from build123d import *

# Parameters (mm, degrees)
BOSS_EXTRUDE1_DEPTH = 15
BOSS_EXTRUDE2_DEPTH = 60
SKETCH3_W           = 30
SKETCH3_H           = 17.5
SKETCH3_H_2         = 34.418211048
CUT_EXTRUDE1_DEPTH  = 199.997487421
BOSS_EXTRUDE3_START = -45
SKETCH4_R           = 5
BOSS_EXTRUDE3_DEPTH = 30


with BuildPart() as part:
    # Sketch1 → Boss-Extrude1 (new body)
    with BuildSketch(Plane(origin=(0, 0, 0), x_dir=(1, 0, 0), z_dir=(0, 1, 0))):
        with BuildLine():
            Line((0, 0), (150, 0))
            Line((150, 0), (150, 60))
            Line((150, 60), (0, 60))
            ThreePointArc((0, 60), (-30, 30), (0, 0))
        make_face()
    extrude(amount=BOSS_EXTRUDE1_DEPTH)

    # Sketch2 → Boss-Extrude2 (add)
    with BuildSketch(Plane.XY):
        with BuildLine():
            Line((60, 15), (90, 15))
            Line((90, 15), (90, 45))
            ThreePointArc((90, 45), (75, 60), (60, 45))
            Line((60, 45), (60, 15))
        make_face()
        with BuildLine():
            Line((120, 15), (150, 15))
            Line((150, 15), (150, 35))
            ThreePointArc((150, 35), (135, 50), (120, 35))
            Line((120, 35), (120, 15))
        make_face()
    extrude(amount=-BOSS_EXTRUDE2_DEPTH)

    # Sketch3 → Cut-Extrude1 (cut, through all)
    with BuildSketch(Plane(origin=(150, 0, 0), x_dir=(0, 0, -1), z_dir=(1, 0, 0))):
        with Locations((30, 26.25)):
            Rectangle(SKETCH3_W, SKETCH3_H)
        with Locations((30, 52.209105524)):
            Rectangle(SKETCH3_W, SKETCH3_H_2)
    extrude(amount=-CUT_EXTRUDE1_DEPTH, mode=Mode.SUBTRACT)

    # Sketch4 → Boss-Extrude3 (add)
    with BuildSketch(Plane.XY.offset(BOSS_EXTRUDE3_START)):
        with Locations(Location((135, 35, 0), (0, 0, 180))):
            Circle(SKETCH4_R)
        with Locations(Location((75, 45, 0), (0, 0, 180))):
            Circle(SKETCH4_R)
    extrude(amount=BOSS_EXTRUDE3_DEPTH)


solid = part.part
Read the model definition and answer for the solid it produces. Units are mm, in the model's axes. A direction names the side the tool comes from. Coordinates: 2 decimals unless noted, no trailing zeros. Write each loop counter-clockwise with the first axis right and the second up, starting at its lowest first coordinate (ties: lowest second). Pieces come first, ordered by that corner, then holes. Notation, with made-up numbers: (59.25, 35.5) -> (113.25, 35.5) arc R14 cw to (113.25, 57.5) -> close; hole circle Ø2 at (-25.75, -22.5). An arc over 180 degrees is marked (long way). Return JSON: item names as keys, results as strings.
(1) The part is cut by section D-D on x = 50. Give the vertices of the cut face in (y, z), then the cut area to 3 significant figures.
Answers below:
{"outline": "(0, -60) -> (15, -60) -> (15, 0) -> (0, 0) -> close", "area": "900 mm^2"}
(2) The part is cut by section B-B on z = -30. Give the vertices of the cut face in (x, y).
Answers below:
{"outline": "(-30, 0) -> (150, 0) -> (150, 17.5) -> (120, 17.5) -> (120, 15) -> (90, 15) -> (90, 17.5) -> (60, 17.5) -> (60, 15) -> (-30, 15) -> close; circle Ø10 at (75, 45); circle Ø10 at (135, 35)"}
(3) For a pull along X with two mould halves and no side action, classify faces 1 (the flat face through (60, 17, -30)), 2 (the cylindrical face through (135, 50, -7)), 3 (the flat face through (139, 30, -45)) as pulls with the +X half, pulls with the -X half, needs draft (parallel to the pull), parting line crosses it, or undercut.
Answers below:
{"face 1": "pulls with the -X half", "face 2": "undercut", "face 3": "needs draft"}
(4) The part is cut by section A-A on x = 75. Give the vertices of the cut face in (y, z), then the cut area to 4 significant figures.
Answers below:
{"outline": "(0, -60) -> (60, -60) -> (60, -45) -> (50, -45) -> (50, -15) -> (60, -15) -> (60, 0) -> (0, 0) -> close; hole (17.5, -45) -> (40, -45) -> (40, -15) -> (17.5, -15) -> close", "area": "2,625 mm^2"}
(5) Consider line 1 along Z through (x, y) = (69.5, 34); line 2 along X through (y, z) = (18.5, -7.5); line 3 along Y through (x, z) = (38, -11). Determine where each line is inside the solid, lowest interval first. Write a range as from..to.
Answers below:
{"line 1": "-60..-45, -15..0", "line 2": "60..90, 120..150", "line 3": "0..15"}
(6) Each of these flat-tipped pins is pushed along its axis until it touches: P1, Ø9, axis at y = 33, z = -33.5, coming from the -X side; P2, Ø8, axis at x = -10.5, y = 11.5, coming from the +Z side; P3, Ø10, axis at y = 6.5, z = -18, coming from the -X side. Where does it stop, or does it pass through?
Answers below:
{"P1": "x = 130", "P2": "z = -0.71", "P3": "x = -29.17"}
(7) The part is cut by section C-C on y = 48. Give the vertices of the cut face in (x, z), then the cut area to 3 significant figures.
Answers below:
{"outline": "(60.3, -60) -> (89.7, -60) -> (89.7, -45) -> (79, -45) -> (79, -15) -> (89.7, -15) -> (89.7, 0) -> (60.3, 0) -> (60.3, -15) -> (71, -15) -> (71, -45) -> (60.3, -45) -> close; (127.52, -60) -> (142.48, -60) -> (142.48, -45) -> (127.52, -45) -> close; (127.52, -15) -> (142.48, -15) -> (142.48, 0) -> (127.52, 0) -> close", "area": "1,570 mm^2"}
(8) Which of the six approach directions +Z, -Z, +X, -X, +Y, -Y give full straight-line access (tool end or side, diameter ignored) to faces 4 (the flat face through (14, 15, -30)), 5 (the flat face through (120, 16, -30)), 6 (the flat face through (135, 17.5, -30)), 7 (the flat face through (132, 30, -15))?
Answers below:
{"face 4": "+Z, -Z, -X, +Y", "face 5": "+Z, -Z, +Y", "face 6": "+X, -X", "face 7": "none"}
